```python
from build123d import *

# Parameters (mm, degrees)
BOSS_EXTRUDE1_DEPTH = 1.5
BOSS_EXTRUDE1_DRAFT = 10
FILLET1_R           = 1


with BuildPart() as part:
    # Sketch2 → Boss-Extrude1 (with draft: the straight prism first)
    with BuildSketch(Plane(origin=(0, 0, 0), x_dir=(1, 0, 0), z_dir=(0, 1, 0))):
        Polygon((15.165421668, 15.165421668), (1.758667474, 8.275044622), (3.841126106, 14.123164889), (-1.358054626, 8.350147449), (-1.358054626, 11.87639847), (-3.626484108, 7.643159543), (-5.804072026, 9.87907884), (-5.982026195, 5.982026195), (-9.87907884, 5.804072026), (-7.643159543, 3.626484108), (-11.87639847, 1.358054626), (-8.350147449, 1.358054626), (-14.123164889, -3.841126106), (-8.275044622, -1.758667474), (-15.165421668, -15.165421668), (-1.758667474, -8.275044622), (-3.841126106, -14.123164889), (1.358054626, -8.350147449), (1.358054626, -11.87639847), (3.626484108, -7.643159543), (5.804072026, -9.87907884), (5.982026195, -5.982026195), (9.87907884, -5.804072026), (7.643159543, -3.626484108), (11.87639847, -1.358054626), (8.350147449, -1.358054626), (14.123164889, 3.841126106), (8.275044622, 1.758667474), align=None)
    extrude(amount=BOSS_EXTRUDE1_DEPTH)
    # Boss-Extrude1: the draft: its side faces are tilted about the plane it starts from
    boss_extrude1_sides = [part.faces().sort_by_distance(p)[0] for p in [
        (8.462044571, 0.75, -11.720233145),
        (2.79989679, 0.75, -11.199104756),
        (1.24153574, 0.75, -11.236656169),
        (-1.358054626, 0.75, -10.11327296),
        (-2.492269367, 0.75, -9.759779007),
        (-4.715278067, 0.75, -8.761119192),
        (-5.893049111, 0.75, -7.930552518),
        (-7.930552518, 0.75, -5.893049111),
        (-8.761119192, 0.75, -4.715278067),
        (-9.759779007, 0.75, -2.492269367),
        (-10.11327296, 0.75, -1.358054626),
        (-11.236656169, 0.75, 1.24153574),
        (-11.199104756, 0.75, 2.79989679),
        (-11.720233145, 0.75, 8.462044571),
        (-8.462044571, 0.75, 11.720233145),
        (-2.79989679, 0.75, 11.199104756),
        (-1.24153574, 0.75, 11.236656169),
        (1.358054626, 0.75, 10.11327296),
        (2.492269367, 0.75, 9.759779007),
        (4.715278067, 0.75, 8.761119192),
        (5.893049111, 0.75, 7.930552518),
        (7.930552518, 0.75, 5.893049111),
        (8.761119192, 0.75, 4.715278067),
        (9.759779007, 0.75, 2.492269367),
        (10.11327296, 0.75, 1.358054626),
        (11.236656169, 0.75, -1.24153574),
        (11.199104756, 0.75, -2.79989679),
        (11.720233145, 0.75, -8.462044571),
    ]]
    draft(boss_extrude1_sides, Plane(origin=(0, 0, 0), x_dir=(1, 0, 0), z_dir=(0, 1, 0)), BOSS_EXTRUDE1_DRAFT)

    # Fillet1
    fillet1_edges = [part.edges().sort_by_distance(p)[0] for p in [
        (7.493053935, 1.5, 5.648260868),
        (8.228576561, 1.5, 4.565827715),
        (9.01135359, 1.5, 2.593250574),
        (9.24203866, 1.5, 1.622545097),
        (10.307546597, 1.5, -0.760721217),
        (10.344144368, 1.5, -2.214694848),
        (11.144016172, 1.5, -7.919500612),
        (7.919500612, 1.5, -11.144016172),
        (2.214694848, 1.5, -10.344144368),
        (0.760721217, 1.5, -10.307546597),
        (4.565827715, 1.5, 8.228576561),
        (-1.622545097, 1.5, -9.24203866),
        (-2.593250574, 1.5, -9.01135359),
        (-4.565827715, 1.5, -8.228576561),
        (-5.648260868, 1.5, -7.493053935),
        (-7.493053935, 1.5, -5.648260868),
        (-8.228576561, 1.5, -4.565827715),
        (-9.01135359, 1.5, -2.593250574),
        (-9.24203866, 1.5, -1.622545097),
        (-10.307546597, 1.5, 0.760721217),
        (-10.344144368, 1.5, 2.214694848),
        (5.648260868, 1.5, 7.493053935),
        (-11.144016172, 1.5, 7.919500612),
        (-7.919500612, 1.5, 11.144016172),
        (-2.214694848, 1.5, 10.344144368),
        (-0.760721217, 1.5, 10.307546597),
        (1.622545097, 1.5, 9.24203866),
        (2.593250574, 1.5, 9.01135359),
    ]]
    fillet(fillet1_edges, radius=FILLET1_R)


solid = part.part
```
Verification items for the finished model (mm, model axes). A direction names the side the tool comes from. Give positions to 0.01 mm unless a question says otherwise; leave off trailing zeros. Order: outer loops, then holes, each group sorted by start corner. A loop starts at its lowest first (then second) coordinate and runs counter-clockwise, first axis right, second up. Notation, with made-up numbers: (60, 47) -> (67, 47) arc R21 cw to (67, 68) -> close; hole circle Ø11 at (-28, 26). An arc over 180 degrees is marked (long way). Use a Markdown table: item, result.
1) Mould release check, pull along Z, two halves, no side actions. Record for faces 1 (the cylindrical face through (7.3, 1.26, 5.47)), 2 (the cylindrical face through (-7.785, 1.26, -4.397)), 3 (the cylindrical face through (0.37, 1.26, -9.59)), 4 (the flat face through (8.68, 0.33, 4.72)): pulls with the +Z half, pulls with the -Z half, needs draft (parallel to the pull), parting line crosses it, or undercut.
Results:
| item | result |
|---|---|
| face 1 | pulls with the +Z half |
| face 2 | undercut |
| face 3 | pulls with the -Z half |
| face 4 | undercut |
2) Tool access check on faces 5 (the cylindrical face through (1.824, 1.26, -9.811)), 6 (the flat face through (-4.685, 0.332, -8.646)), 7 (the cylindrical face through (-9.69, 1.26, 0.46)), 8 (the cylindrical face through (-0.37, 1.26, 9.59)), 9 (the cylindrical face through (9.69, 1.26, -0.46)). Record the directions out of +Z, -Z, +X, -X, +Y, -Y that give a thin tool (end or side, any length) a straight path to the whole face; none if there is none.
Results:
| item | result |
|---|---|
| face 5 | +Y |
| face 6 | -Z, +Y |
| face 7 | -X, +Y |
| face 8 | +Z, +Y |
| face 9 | +X, +Y |
3) Depth check by flat-ended pin: pin 1 Ø1.5 at (x, z) = (-9, -0.5) entering from +Y; pin 2 Ø6 at (x, z) = (10, -1) entering from -Y. Enter the tip coordinate at first touch or a pass-through.
Results:
| item | result |
|---|---|
| pin 1 | y = 1.49 |
| pin 2 | y = 0 |
4) Section check A-A, the plane y = 0.4. Record the boundary of the cut face in (x, z).
Results:
| item | result |
|---|---|
| outline | (-15, 15) -> (-8.13, 1.63) -> (-13.81, 3.66) -> (-8.17, -1.43) -> (-11.6, -1.43) -> (-7.52, -3.61) -> (-9.71, -5.74) -> (-5.91, -5.91) -> (-5.74, -9.71) -> (-3.61, -7.52) -> (-1.43, -11.6) -> (-1.43, -8.17) -> (3.66, -13.81) -> (1.63, -8.13) -> (15, -15) -> (8.13, -1.63) -> (13.81, -3.66) -> (8.17, 1.43) -> (11.6, 1.43) -> (7.52, 3.61) -> (9.71, 5.74) -> (5.91, 5.91) -> (5.74, 9.71) -> (3.61, 7.52) -> (1.43, 11.6) -> (1.43, 8.17) -> (-3.66, 13.81) -> (-1.63, 8.13) -> close |
5) Section check B-B, the plane x = -11. Give the number of separate pieces and of enclosed holes in the cut face, then the cut area to 3 significant figures.
Results:
| item | result |
|---|---|
| separate pieces | 3 |
| enclosed holes | 0 |
| area | 9.85 mm² |
6) Material ranges on probe 1 along Z at (x, y) = (-10, 1.1); probe 2 along X at (y, z) = (0.2, 10); probe 3 along X at (y, z) = (0.6, 10), recorded low to high.
Results:
| item | result |
|---|---|
| probe 1 | -2.02 to -1.66, 0.54 to 2.05, 5.78 to 12.17 |
| probe 2 | -12.47 to -5.19, -2.34 to -0.18, 1.39 to 2.32 |
| probe 3 | -12.39 to -5.35, -2.26 to -0.27, 1.46 to 2.24 |
